For this review, take the finished solid that the model builds, in its own axes (mm). Face numbers are marked on the shaded views. Round coordinates to 2 decimals unless told otherwise and drop trailing zeros. Order: outer loops, then holes, each group sorted by start corner. A loop starts at its lowest first (then second) coordinate and runs counter-clockwise, first axis right, second up. Notation, with made-up numbers: M 34,72.25 L 42,72.25 A20 cw 42,84.25 Z; hole C 89.5,47.25 d2. An arc over 180 degrees is marked long. Answer as a JSON object with one key per item and string values.
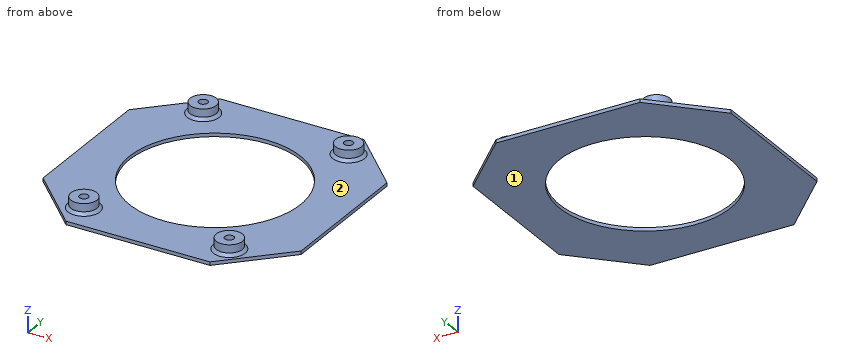
from build123d import *

# Parameters (mm, degrees)
SKETCH2_W           = 90.475
SKETCH2_H           = 1.2
BOSS_EXTRUDE1_DEPTH = 90.475
SKETCH3_R           = 4.587496825
SKETCH3_R_2         = 1.587496825
EXTRUDE_THIN1_DEPTH = 3.8
CHAMFER1_SIZE       = 1
SKETCH5_R           = 30
CUT_EXTRUDE1_DEPTH  = 106.553838455
CHAMFER2_SIZE       = 20


with BuildPart() as part:
    # Sketch2 → Boss-Extrude1 (new body)
    with BuildSketch(Plane(origin=(0, 4.7625, 0), x_dir=(1, 0, 0), z_dir=(0, 1, 0))):
        with Locations((0, -0.6)):
            Rectangle(SKETCH2_W, SKETCH2_H)
    extrude(amount=BOSS_EXTRUDE1_DEPTH)

    # Sketch3 → Extrude-Thin1 (add)
    # profile 1 of 4: a face of its own
    with BuildSketch(Plane(origin=(0, 0, 5), x_dir=(-1, 0, 0), z_dir=(0, 0, -1))):
        with Locations((25.003889322, 84.960201446)):
            Circle(SKETCH3_R)
        with Locations((25.003889322, 84.960201446)):
            Circle(SKETCH3_R_2, mode=Mode.SUBTRACT)
    # profile 2 of 4: a face of its own
    with BuildSketch(Plane(origin=(0, 0, 5), x_dir=(-1, 0, 0), z_dir=(0, 0, -1))):
        with Locations((-25.995997859, 84.926982308)):
            Circle(SKETCH3_R)
        with Locations((-25.995997859, 84.926982308)):
            Circle(SKETCH3_R_2, mode=Mode.SUBTRACT)
    # profile 3 of 4: a face of its own
    with BuildSketch(Plane(origin=(0, 0, 5), x_dir=(-1, 0, 0), z_dir=(0, 0, -1))):
        with Locations((25.049484218, 14.960356296)):
            Circle(SKETCH3_R)
        with Locations((25.049484218, 14.960356296)):
            Circle(SKETCH3_R_2, mode=Mode.SUBTRACT)
    # profile 4 of 4: a face of its own
    with BuildSketch(Plane(origin=(0, 0, 5), x_dir=(-1, 0, 0), z_dir=(0, 0, -1))):
        with Locations((-25.950402964, 14.927137158)):
            Circle(SKETCH3_R)
        with Locations((-25.950402964, 14.927137158)):
            Circle(SKETCH3_R_2, mode=Mode.SUBTRACT)
    extrude(amount=EXTRUDE_THIN1_DEPTH)

    # Chamfer1
    chamfer1_edges = [part.edges().sort_by_distance(p)[0] for p in [
        (-20.416392497, 84.960201446, 1.2),
        (30.583494684, 84.926982308, 1.2),
        (-20.461987393, 14.960356296, 1.2),
        (30.537899789, 14.927137158, 1.2),
    ]]
    chamfer(chamfer1_edges, length=CHAMFER1_SIZE)

    # Sketch5 → Cut-Extrude1 (cut, through all)
    with BuildSketch(Plane(origin=(0, 0, 0), x_dir=(-1, 0, 0), z_dir=(0, 0, -1))):
        with Locations((0, 50)):
            Circle(SKETCH5_R)
    extrude(amount=-CUT_EXTRUDE1_DEPTH, mode=Mode.SUBTRACT)

    # Chamfer2
    chamfer2_edges = [part.edges().sort_by_distance(p)[0] for p in [
        (-45.2375, 95.2375, 0.6),
        (45.2375, 95.2375, 0.6),
        (-45.2375, 4.7625, 0.6),
        (45.2375, 4.7625, 0.6),
    ]]
    chamfer(chamfer2_edges, length=CHAMFER2_SIZE)


solid = part.part
1) Add section A-A on x = 0. State the section outline as (y, z) points, and give its area (3 significant figures).
Geometry check:
{"outline": "M 4.76,0 L 20,0 L 20,1.2 L 4.76,1.2 Z; M 80,0 L 95.24,0 L 95.24,1.2 L 80,1.2 Z", "area": "36.6 mm²"}
2) Mouldability with a two-part tool opening along Y and no side actions: class the marked faces 1 and 2 as +Y half, -Y half, draft (parallel to the pull), parting line (faces both ways), or undercut.
Geometry check:
{"face 1": "draft", "face 2": "undercut"}
3) Add section B-B on y = 50. State the section outline as (x, z) points.
Geometry check:
{"outline": "M -45.24,0 L -30,0 L -30,1.2 L -45.24,1.2 Z; M 30,0 L 45.24,0 L 45.24,1.2 L 30,1.2 Z"}
4) Add section C-C on z = 4.15. State the section outline as (x, y) points (1 decimal).
Geometry check:
{"outline": "C -25,15 d9.2; C -25,85 d9.2; C 26,14.9 d9.2; C 26,84.9 d9.2; hole C -25,15 d3.2; hole C -25,85 d3.2; hole C 26,14.9 d3.2; hole C 26,84.9 d3.2"}
5) Insertion check: P1, Ø1, axis at x = -26, y = 15, coming from the +Z side; P2, Ø3, axis at y = 77, z = 1.5, coming from the -X side. Each pin has a flat end and moves straight along its axis. Give the tip position at first contact, or say it passes through.
Geometry check:
{"P1": "stops at z = 1.2", "P2": "stops at x = -44.94"}
6) For L1, parallel to X at y = 85, z = 4.3; L2, parallel to Y at x = 0, z = 0.95; L3, parallel to Z at x = 35, y = 83, list the stretches that pass through material, from the lowest coordinate up.
Geometry check:
{"L1": "x = -29.59 to -26.59, -23.42 to -20.42, 21.41 to 24.41, 27.58 to 30.58", "L2": "y = 4.76 to 20, 80 to 95.24", "L3": "z = 0 to 1.2"}
